Geometry check sheet. Reference: drawing and pictorial views, mm from the part's lowest x, y, z. Give positions to 0.01 mm unless a question says otherwise; leave off trailing zeros. Order: outer loops, then holes, each group sorted by start corner. A loop starts at its lowest first (then second) coordinate and runs counter-clockwise, first axis right, second up.
Item 1: Sectioned sample at B-B on y = 2.25. Record the boundary of the cut face in (x, z), and give its area (3 significant figures).
Item 2: Release check for a two-part mould opening along Y. For the marked faces 1 and 2 record: released by +Y, released by -Y, zero draft, split by the parting line, or undercut.
Item 3: Material ranges on line 1 along X through (y, z) = (7.5, 125.75); line 2 along Y through (x, z) = (25, 126.75); line 3 along X through (y, z) = (1.5, 5), recorded low to high.
Item 4: Gauge pin test, flat ends, axial feed: P1, Ø7.5, axis at x = 131.5, y = 6.5, coming from the -Z side; P2, Ø3.5, axis at x = 25, y = 7.5, coming from the +Z side; P3, Ø6, axis at x = 224, y = 12.5, coming from the -Z side. Record the tip position at first contact, or that the pin passes through.
Item 5: Sectioned sample at A-A on z = 27.5. Record the boundary of the cut face in (x, y).
Item 6: Sectioned sample at C-C on x = 191.5. Record the boundary of the cut face in (y, z), and give its area (3 significant figures).
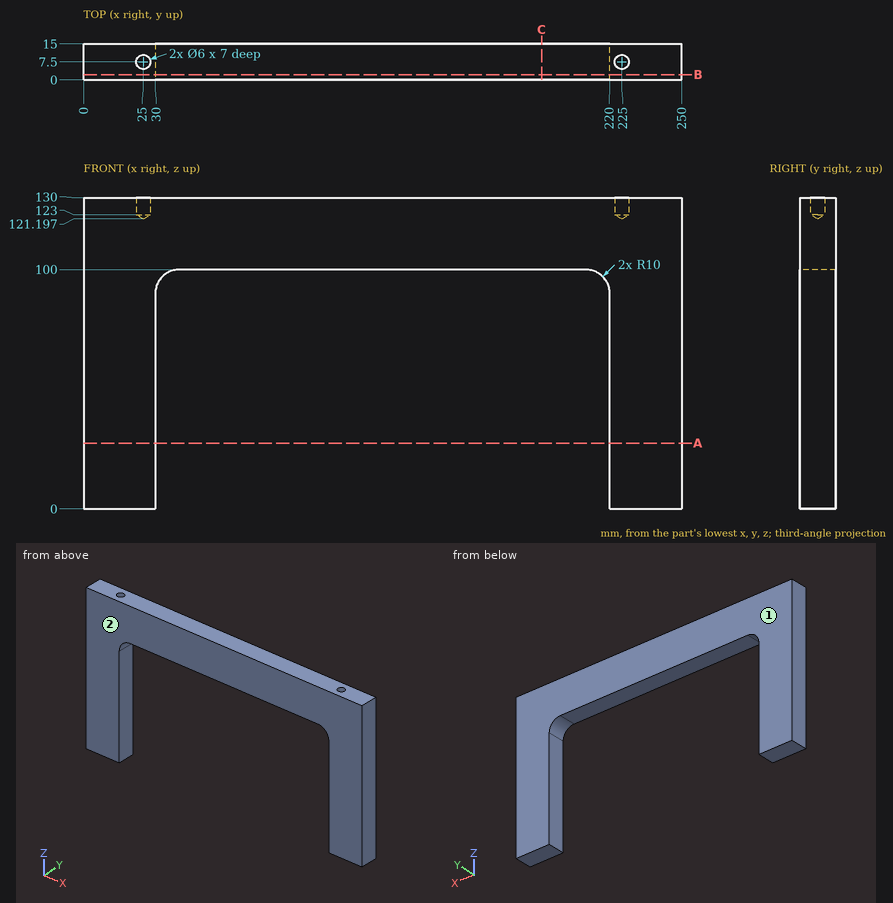
Report:
1. outline: (0, 0) - (30, 0) - (30, 90) arc R10 cw to (40, 100) - (210, 100) arc R10 cw to (220, 90) - (220, 0) - (250, 0) - (250, 130) - (0, 130) - close
1. area: 13,500 mm2
2. face 1: released by +Y
2. face 2: released by -Y
3. line 1: x = 0 to 22, 28 to 222, 228 to 250
3. line 2: y = 0 to 4.5, 10.5 to 15
3. line 3: x = 0 to 30, 220 to 250
4. P1: stops at z = 100
4. P2: stops at z = 122.25
4. P3: stops at z = 0
5. outline: (0, 0) - (30, 0) - (30, 15) - (0, 15) - close; (220, 0) - (250, 0) - (250, 15) - (220, 15) - close
6. outline: (0, 100) - (15, 100) - (15, 130) - (0, 130) - close
6. area: 450 mm2
